Here's how the part is built. I have some questions about the finished solid (model axes, mm). Face numbers are marked on the shaded views. A direction names the side the tool comes from. Round coordinates to 2 decimals unless told otherwise and drop trailing zeros. Write each loop counter-clockwise with the first axis right and the second up, starting at its lowest first coordinate (ties: lowest second). Pieces come first, ordered by that corner, then holes. Notation, with made-up numbers: M -6,43 L 20,43 A20 cw 20,61 Z; hole C 19,37.25 d4. An arc over 180 degrees is marked long. Write item = value, one per line. Start each with the question number.
(1) I want a section at C-C (x = -1). List the corners of the cut face in (y, z) for me, and give its area (3 significant figures).
(2) I need wall thicknesses on line 1 along Z through (x, y) = (-12.5, 0.95) (3 decimals); line 2 along X through (y, z) = (4.3, -6.55); line 3 along X through (y, z) = (2.1, -6.55). Which ranges of each line are inside material? Lowest first, please.
(3) Will this pin go through, and if not, where does the flat tip stop? pin 1 Ø4 at (x, z) = (11.1, 6.55) entering from -Y.
(4) If we mould it in two halves opening along Z, with no side actions, what happens to the marked faces 1, 2, 3 and 4? For each: released by +Z, released by -Z, zero draft, split by the parting line, or undercut.
(5) On a 3-axis mill with a long thin cutter (end or side, diameter ignored), from which of +Z, -Z, +X, -X, +Y, -Y can I reach the whole of each face in a straight line? I mean the marked faces 5 and 6. Say none if no direction works.
(6) I want a section at A-A (x = 11.1). Give the number of separate pieces and of enclosed holes in the cut face, and give its area (3 significant figures).
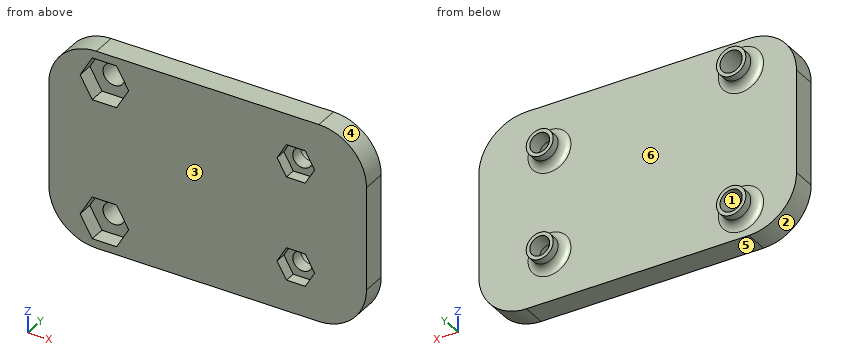
```python
from build123d import *

# Parameters (mm, degrees)
SKETCH1_W           = 40
SKETCH1_H           = 25
SKETCH1_R           = 1.4
BOSS_EXTRUDE1_DEPTH = 3
SKETCH2_R           = 1.25
CUT_EXTRUDE1_DEPTH  = 24.774986856
SKETCH4_R           = 1.85
SKETCH4_R_2         = 1.4
SKETCH4_R_3         = 1.7
SKETCH4_R_4         = 1.25
BOSS_EXTRUDE2_DEPTH = 2
FILLET1_R           = 1
CUT_EXTRUDE2_DEPTH  = 2
CUT_EXTRUDE3_DEPTH  = 1.4
FILLET2_R           = 6


with BuildPart() as part:
    # Sketch1 → Boss-Extrude1 (new body)
    with BuildSketch(Plane(origin=(0, 0, 0), x_dir=(1, 0, 0), z_dir=(0, 1, 0))):
        Rectangle(SKETCH1_W, SKETCH1_H)
        with Locations(Location((-13, 8.825, 0), (0, 0, 270))):
            Circle(SKETCH1_R, mode=Mode.SUBTRACT)
        with Locations(Location((-13, -8.825, 0), (0, 0, 270))):
            Circle(SKETCH1_R, mode=Mode.SUBTRACT)
    extrude(amount=BOSS_EXTRUDE1_DEPTH)

    # Sketch2 → Cut-Extrude1 (cut, through all)
    with BuildSketch(Plane(origin=(0, 3, 0), x_dir=(1, 0, 0), z_dir=(0, 1, 0))):
        with Locations(Location((11.1, 6.55, 0), (0, 0, 270))):
            Circle(SKETCH2_R)
        with Locations(Location((11.1, -6.55, 0), (0, 0, 90))):
            Circle(SKETCH2_R)
    extrude(amount=-CUT_EXTRUDE1_DEPTH, mode=Mode.SUBTRACT)

    # Sketch4 → Boss-Extrude2 (add)
    # profile 1 of 4: a face of its own
    with BuildSketch(Plane(origin=(0, 3, 0), x_dir=(1, 0, 0), z_dir=(0, 1, 0))):
        with Locations(Location((-13, 8.825, 0), (0, 0, 270))):
            Circle(SKETCH4_R)
        with Locations(Location((-13, 8.825, 0), (0, 0, 270))):
            Circle(SKETCH4_R_2, mode=Mode.SUBTRACT)
    # profile 2 of 4: a face of its own
    with BuildSketch(Plane(origin=(0, 3, 0), x_dir=(1, 0, 0), z_dir=(0, 1, 0))):
        with Locations(Location((11.1, 6.55, 0), (0, 0, 270))):
            Circle(SKETCH4_R_3)
        with Locations(Location((11.1, 6.55, 0), (0, 0, 270))):
            Circle(SKETCH4_R_4, mode=Mode.SUBTRACT)
    # profile 3 of 4: a face of its own
    with BuildSketch(Plane(origin=(0, 3, 0), x_dir=(1, 0, 0), z_dir=(0, 1, 0))):
        with Locations(Location((11.1, -6.55, 0), (0, 0, 270))):
            Circle(SKETCH4_R_3)
        with Locations(Location((11.1, -6.55, 0), (0, 0, 270))):
            Circle(SKETCH4_R_4, mode=Mode.SUBTRACT)
    # profile 4 of 4: a face of its own
    with BuildSketch(Plane(origin=(0, 3, 0), x_dir=(1, 0, 0), z_dir=(0, 1, 0))):
        with Locations(Location((-13, -8.825, 0), (0, 0, 270))):
            Circle(SKETCH4_R)
        with Locations(Location((-13, -8.825, 0), (0, 0, 270))):
            Circle(SKETCH4_R_2, mode=Mode.SUBTRACT)
    extrude(amount=BOSS_EXTRUDE2_DEPTH)

    # Fillet1
    fillet1_edges = [part.edges().sort_by_distance(p)[0] for p in [
        (-13, 3, -10.675),
        (11.1, 3, -8.25),
        (11.1, 3, 4.85),
        (-13, 3, 6.975),
    ]]
    fillet(fillet1_edges, radius=FILLET1_R)

    # Sketch5 → Cut-Extrude2 (cut)
    with BuildSketch(Plane.XZ):
        Polygon((-11.470021787, 6.175), (-9.940043573, 8.825), (-11.470021787, 11.475), (-14.529978213, 11.475), (-16.059956427, 8.825), (-14.529978213, 6.175), align=None)
        Polygon((-11.470021787, -11.475), (-9.940043573, -8.825), (-11.470021787, -6.175), (-14.529978213, -6.175), (-16.059956427, -8.825), (-14.529978213, -11.475), align=None)
    extrude(amount=-CUT_EXTRUDE2_DEPTH, mode=Mode.SUBTRACT)

    # Sketch6 → Cut-Extrude3 (cut)
    with BuildSketch(Plane.XZ):
        Polygon((12.283568052, 4.5), (13.467136104, 6.55), (12.283568052, 8.6), (9.916431948, 8.6), (8.732863896, 6.55), (9.916431948, 4.5), align=None)
        Polygon((12.283568052, -8.6), (13.467136104, -6.55), (12.283568052, -4.5), (9.916431948, -4.5), (8.732863896, -6.55), (9.916431948, -8.6), align=None)
    extrude(amount=-CUT_EXTRUDE3_DEPTH, mode=Mode.SUBTRACT)

    # Fillet2
    fillet2_edges = [part.edges().sort_by_distance(p)[0] for p in [
        (-20, 1.5, -12.5),
        (20, 1.5, -12.5),
        (20, 1.5, 12.5),
        (-20, 1.5, 12.5),
    ]]
    fillet(fillet2_edges, radius=FILLET2_R)


solid = part.part
```
Returned:
q1.outline = M 0,-12.5 L 3,-12.5 L 3,12.5 L 0,12.5 Z
q1.area = 75.0 mm²
q2.line_1 = -12.5 to -11.475, -6.175 to 6.175, 11.475 to 12.5
q2.line_2 = 9.4 to 9.85, 12.35 to 12.8
q2.line_3 = -20 to 9.85, 12.35 to 20
q3.pin_1 = 1.4
q4.face_1 = undercut
q4.face_2 = released by -Z
q4.face_3 = zero draft
q4.face_4 = released by +Z
q5.face_5 = -Z, +X, -X, +Y, -Y
q5.face_6 = +Y
q6.separate_pieces = 3
q6.enclosed_holes = 0
q6.area = 60.0 mm²
